from build123d import *

# Parameters (mm, degrees)
F0_W     = 250
F0_H     = 300
F1_DEPTH = 25
F2_W     = 25
F2_H     = 300
F3_DEPTH = 25
F4_R     = 5
F5_DEPTH = 25


with BuildPart() as f1:
    # F0 (on Right) → F1 (new body)
    with BuildSketch(Plane.YZ):
        Rectangle(F0_W, F0_H)
    extrude(amount=F1_DEPTH)

    # F2 (on face) → F3 (join)
    with BuildSketch(Plane.YZ.offset(25)):
        with Locations((-62.5, 0)):
            Rectangle(F2_W, F2_H)
        with Locations((12.5, 0)):
            Rectangle(F2_W, F2_H)
    extrude(amount=F3_DEPTH)

    # F4 (on face) → F5 (cut, through all)
    with BuildSketch(Plane.YZ.offset(25)):
        with Locations((86.464388, 120)):
            Circle(F4_R)
        with Locations((38.535612, 68.982038)):
            Circle(F4_R)
        with Locations((38.535612, 120)):
            Circle(F4_R)
        with Locations((86.464388, 68.982038)):
            Circle(F4_R)
        with Locations((86.464388, -68.982038)):
            Circle(F4_R)
        with Locations((86.464388, -120)):
            Circle(F4_R)
        with Locations((38.535612, -120)):
            Circle(F4_R)
        with Locations((38.535612, -68.982038)):
            Circle(F4_R)
    extrude(amount=-F5_DEPTH, mode=Mode.SUBTRACT)


solid = f1.part
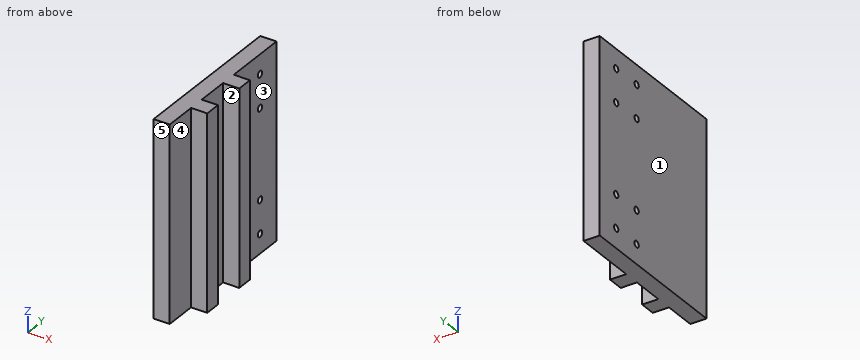
Geometry check sheet. Reference: the model listing, model coordinates, mm. Face numbers are marked on the shaded views. A direction names the side the tool comes from. Round coordinates to 2 decimals unless told otherwise and drop trailing zeros. Loops run counter-clockwise (first coordinate to the right, second up) from the corner with the lowest first, then second, coordinate; pieces in that order, holes last. Notation, with made-up numbers: (80.5, 14) -> (114.5, 14) arc R17 cw to (114.5, 34) -> close; hole circle Ø1 at (-20, 66.5). An arc over 180 degrees is marked (long way). Answer as a JSON object with one key per item and string values. Group by question number.
Item 1: Thickness scan on line 1 along Y through (x, z) = (35.5, -66); line 2 along Y through (x, z) = (2.5, 121.5); line 3 along Y through (x, z) = (3, 65.5). Record the ranges inside material, lowest first.
Item 2: Cross-section at D-D, the plane y = 69. Record the cut outline in (x, z), plus the area to 3 significant figures.
Item 3: Set-up check for the marked faces 1, 2, 3, 4 and 5: record each of +Z, -Z, +X, -X, +Y, -Y from which the full face is reachable in a straight line by a thin tool's end or side.
Item 4: Cross-section at A-A, the plane z = -120. Record the cut outline in (x, y), plus the area to 3 significant figures.
Item 5: Depth check by flat-ended pin: pin 1 Ø11.5 at (y, z) = (86.46, 68.98) entering from +X; pin 2 Ø12.5 at (x, z) = (41, -23.5) entering from -Y; pin 3 Ø7.5 at (x, z) = (40, -30.5) entering from +Y. Enter the tip coordinate at first touch or a pass-through.
Item 6: Cross-section at B-B, the plane x = 35. Record the cut outline in (y, z), plus the area to 3 significant figures.
Item 7: Cross-section at C-C, the plane y = 40. Record the cut outline in (x, z).
Determined:
{
 "1": {"line 1": "y = -75 to -50, 0 to 25", "line 2": "y = -125 to 33.77, 43.31 to 81.69, 91.23 to 125", "line 3": "y = -125 to 34.95, 42.12 to 82.88, 90.05 to 125"},
 "2": {"outline": "(0, -150) -> (25, -150) -> (25, 150) -> (0, 150) -> close", "area": "7,500 mm²"},
 "3": {"face 1": "+Z, -Z, -X, +Y, -Y", "face 2": "+Z, -Z, +X", "face 3": "+Z, -Z, +X, +Y", "face 4": "+Z, -Z, +X, -Y", "face 5": "+Z, -Z, +X, -X, -Y"},
 "4": {"outline": "(0, -125) -> (25, -125) -> (25, -75) -> (50, -75) -> (50, -50) -> (25, -50) -> (25, 0) -> (50, 0) -> (50, 25) -> (25, 25) -> (25, 33.54) -> (0, 33.54) -> close; (0, 43.54) -> (25, 43.54) -> (25, 81.46) -> (0, 81.46) -> close; (0, 91.46) -> (25, 91.46) -> (25, 125) -> (0, 125) -> close", "area": "7,000 mm²"},
 "5": {"pin 1": "stops at x = 25", "pin 2": "stops at y = -75", "pin 3": "stops at y = 25"},
 "6": {"outline": "(-75, -150) -> (-50, -150) -> (-50, 150) -> (-75, 150) -> close; (0, -150) -> (25, -150) -> (25, 150) -> (0, 150) -> close", "area": "15,000 mm²"},
 "7": {"outline": "(0, -150) -> (25, -150) -> (25, -124.78) -> (0, -124.78) -> close; (0, -115.22) -> (25, -115.22) -> (25, -73.76) -> (0, -73.76) -> close; (0, -64.2) -> (25, -64.2) -> (25, 64.2) -> (0, 64.2) -> close; (0, 73.76) -> (25, 73.76) -> (25, 115.22) -> (0, 115.22) -> close; (0, 124.78) -> (25, 124.78) -> (25, 150) -> (0, 150) -> close"}
}
